Autodesk Inventor part; units mm, degrees
ref_plane "YZ Plane" through (0, 0, 0) normal (1, 0, 0) x (0, 1, 0)
ref_plane "XZ Plane" through (0, 0, 0) normal (0, 1, 0) x (-1, 0, 0)
ref_plane "XY Plane" through (0, 0, 0) normal (0, 0, 1) x (1, 0, 0)
sketch "Sketch1" plane through (0, 0, 0) normal (0, 0, 1) x (1, 0, 0)
  circle A0 centre (0, 0) radius 5
  dimension "d0" = 10
extrude "Extrusion1" add sketch "Sketch1" along normal blind 30 draft -3
sketch "Sketch2" plane through (0, 0, 30) normal (0, 0, 1) x (1, 0, 0)
  circle A0 centre (0, 0) radius 2.8754
extrude "Extrusion2" add sketch "Sketch2" along normal blind 5
fillet "Fillet1" radius 2 1 edges at (-2.8754, 0, 35)
sketch "Sketch3" plane through (0, 0, 0) normal (1, 0, 0) x (0, 1, 0)
  circle A0 centre (0, 31.6406) radius 1.6406
  line L0 (-2.8754, 30) -> (2.8754, 30)
  point P0 (0, 0)
extrude "Extrusion3" cut sketch "Sketch3" along normal through all both and the other way through all
properties part number "arms"
CAD build for the part. Positions are in the model's coordinates, mm. A direction names the side the tool comes from. Coordinates: 2 decimals unless noted, no trailing zeros. Order: outer loops, then holes, each group sorted by start corner. A loop starts at its lowest first (then second) coordinate and runs counter-clockwise, first axis right, second up. Notation, with made-up numbers: (21, 37.25) -> (66, 37.25) arc R3 ccw to (66, 42.25) -> close; hole circle Ø5 at (59.5, -28). An arc over 180 degrees is marked (long way). Answer in a Markdown table with one row per item.
1) Drill centre lines: line 1 (Z direction, x = -0.9, y = 0); line 2 (Z direction, x = -0.5, y = -1); line 3 (X direction, y = -3.5, z = 9). Where is each one in solid material? Low to high.
Check values:
| item | result |
|---|---|
| line 1 | 0 to 30, 33.28 to 35 |
| line 2 | 0 to 30.34, 32.94 to 34.99 |
| line 3 | -2.87 to 2.87 |
2) Which spindle directions (+Z, -Z, +X, -X, +Y, -Y) get a long thin tool onto all of the face, cutting with end or side? Do faces 1 (the face through (-0.063, 2.875, 31.479)), 2 (the face through (-1, 3, 30)), 3 (the face through (0.063, -2.875, 31.479)). Say none if no direction does.
Check values:
| item | result |
|---|---|
| face 1 | +Z, +Y |
| face 2 | +Z |
| face 3 | +Z, -Y |
3) Band-saw the part on B-B (z = 2.5). List the corners of the cut face in (x, y), and give its area (3 significant figures).
Check values:
| item | result |
|---|---|
| outline | circle Ø9.74 at (0, 0) |
| area | 74.5 mm2 |
4) Mould opens along Z. For faces 4 (the face through (-0.916, 4.124, 14.79)), 5 (the face through (0, 0, 0)), 6 (the face through (-0.04, -1.21, 30.53)) say: pulls with the +Z half, pulls with the -Z half, needs draft (parallel to the pull), parting line crosses it, or undercut.
Check values:
| item | result |
|---|---|
| face 4 | pulls with the +Z half |
| face 5 | pulls with the -Z half |
| face 6 | undercut |
5) Band-saw the part on A-A (z = 29.5). List the corners of the cut face in (x, y).
Check values:
| item | result |
|---|---|
| outline | circle Ø6.91 at (0, 0) |
6) Flat gauge pins, fed straight in: P1, Ø5, axis at x = -4, z = 23, coming from the +Y side; P2, Ø3, axis at y = -0.5, z = 22.5, coming from the -X side. Where does each tip first touch, or does it go through?
Check values:
| item | result |
|---|---|
| P1 | y = 3.49 |
| P2 | x = -3.9 |
